Source: CAD feature listing. Evaluate the final solid. Frame: model axes, mm. Face numbers are marked on the shaded views. A direction names the side the tool comes from. Coordinates: 2 decimals unless noted, no trailing zeros. Write each loop counter-clockwise with the first axis right and the second up, starting at its lowest first coordinate (ties: lowest second). Pieces come first, ordered by that corner, then holes. Notation, with made-up numbers: M 63.5,39.5 L 73.5,39.5 A27 ccw 73.5,69.5 Z; hole C 54,-31.75 d1. An arc over 180 degrees is marked long. One line per item, written item: value. Start each with the question number.
Item 1: Pin query (flat end, axial travel): P1, Ø4, axis at y = 33.5, z = -35.5, coming from the -X side; P2, Ø1.5, axis at x = -26, z = -5, coming from the +Y side; P3, Ø20, axis at x = 27.5, y = 32, coming from the +Z side. Return the tip coordinate at first contact, or that it passes through.
Item 2: Cut plane B-B, the plane z = -35.86. Output: boundary loops of the cut face in (x, y).
Item 3: Set-up query: the marked faces 1 and 2. Return all of +Z, -Z, +X, -X, +Y, -Y with unobstructed straight access to the full face (end or side cutting, diameter ignored); none if empty.
Item 4: Cut plane A-A, the plane y = 34.35. Output: boundary loops of the cut face in (x, z), then the cut area to 3 significant figures.
Item 5: Cut plane C-C, the plane x = 27. Output: boundary loops of the cut face in (y, z), then the cut area to 3 significant figures.
Item 6: Cut plane D-D, the plane x = -11. Output: boundary loops of the cut face in (y, z), then the cut area to 3 significant figures.
Item 7: Ray query, L1, parallel to Y at x = -17.5, z = 32.5; L2, parallel to Z at x = 18, y = 33.5; L3, parallel to X at y = 6.5, z = -38. Return the intervals inside material, ascending. Write a range as from..to.
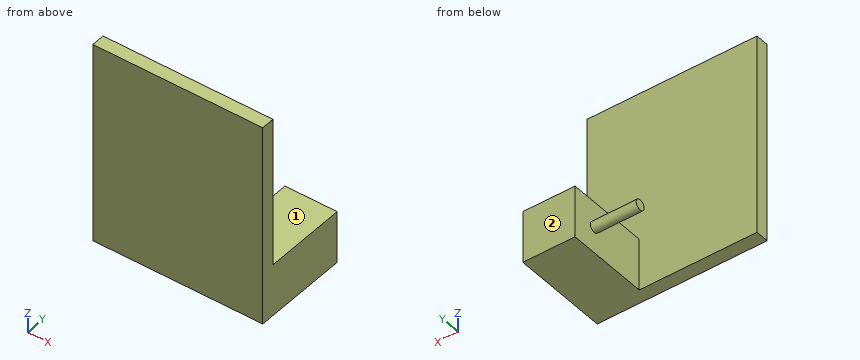
```python
from build123d import *

# Parameters (mm, degrees)
SKETCH1_W           = 81.4
SKETCH1_H           = 96.72
BOSS_EXTRUDE1_DEPTH = 6.35
SKETCH2_W           = 25
SKETCH2_H           = 25
BOSS_EXTRUDE2_DEPTH = 40
SKETCH3_R           = 2.5
BOSS_EXTRUDE3_DEPTH = 22


with BuildPart() as part:
    # Sketch1 → Boss-Extrude1 (new body)
    with BuildSketch(Plane(origin=(0, 0, 0), x_dir=(1, 0, 0), z_dir=(0, 1, 0))):
        Rectangle(SKETCH1_W, SKETCH1_H)
    extrude(amount=BOSS_EXTRUDE1_DEPTH)

    # Sketch2 → Boss-Extrude2 (add)
    with BuildSketch(Plane(origin=(0, 6.35, 0), x_dir=(1, 0, 0), z_dir=(0, 1, 0))):
        with Locations((28.2, 35.86)):
            Rectangle(SKETCH2_W, SKETCH2_H)
    extrude(amount=BOSS_EXTRUDE2_DEPTH)

    # Sketch3 → Boss-Extrude3 (add)
    with BuildSketch(Plane.ZY.offset(-15.7)):
        with Locations(Location((-35.86, 34.35, 0), (0, 0, 180))):
            Circle(SKETCH3_R)
    extrude(amount=BOSS_EXTRUDE3_DEPTH)


solid = part.part
```
From the geometry:
1. P1: stops at x = -6.3
1. P2: stops at y = 6.35
1. P3: stops at z = -23.36
2. outline: M -40.7,0 L 40.7,0 L 40.7,46.35 L 15.7,46.35 L 15.7,36.85 L -6.3,36.85 L -6.3,31.85 L 15.7,31.85 L 15.7,6.35 L -40.7,6.35 Z
3. face 1: +Z, +X, -X, +Y
3. face 2: +Z, -Z, +X, -X, +Y
4. outline: M -6.3,-38.36 L 15.7,-38.36 L 15.7,-48.36 L 40.7,-48.36 L 40.7,-23.36 L 15.7,-23.36 L 15.7,-33.36 L -6.3,-33.36 Z
4. area: 735 mm²
5. outline: M 0,-48.36 L 46.35,-48.36 L 46.35,-23.36 L 6.35,-23.36 L 6.35,48.36 L 0,48.36 Z
5. area: 1,610 mm²
6. outline: M 0,-48.36 L 6.35,-48.36 L 6.35,48.36 L 0,48.36 Z
6. area: 614 mm²
7. L1: y = 0..6.35
7. L2: z = -48.36..-23.36
7. L3: x = 15.7..40.7
